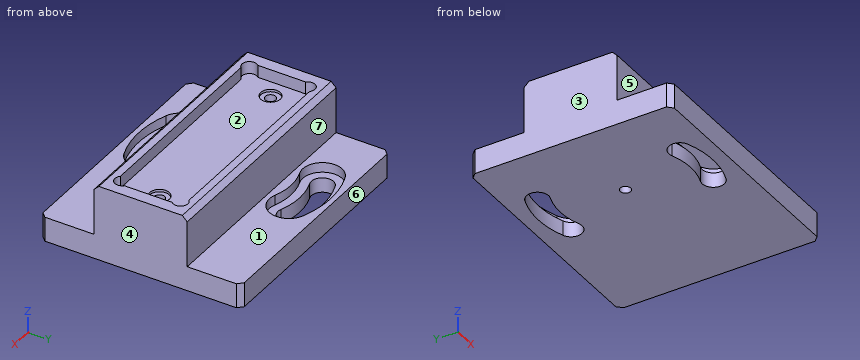
Autodesk Inventor part; units mm, degrees
ref_plane "YZ Plane" through (0, 0, 0) normal (1, 0, 0) x (0, 1, 0)
ref_plane "XZ Plane" through (0, 0, 0) normal (0, 1, 0) x (-1, 0, 0)
ref_plane "XY Plane" through (0, 0, 0) normal (0, 0, 1) x (1, 0, 0)
sketch "Sketch1" plane through (0, 0, 0) normal (0, 0, 1) x (1, 0, 0)
  line L0 (-24.4, -9.5) -> (24.4, -9.5)
  line L1 (24.4, -9.5) -> (24.4, 9.5)
  line L2 (24.4, 9.5) -> (-24.4, 9.5)
  line L3 (-24.4, 9.5) -> (-24.4, -9.5)
  line L4 (-24.4, -9.5) -> (24.4, 9.5) construction
  line L5 (24.4, -9.5) -> (-24.4, 9.5) construction
  point P0 (0, 0)
  dimension "LENGTH" = 48.8
  dimension "WIDTH" = 19
extrude "Extrusion1" add sketch "Sketch1" along normal blind 12.85
sketch "Sketch2" plane through (0, 0, 12.85) normal (0, 0, 1) x (1, 0, 0)
  point P0 (0, 0)
  point P1 (-18.2, 0)
  point P2 (18.2, 0)
  dimension "d11" = 0
  dimension "d12" = 0
  dimension "d13" = 36.4
  dimension "d14" = 18.2
hole "Hole1" at (-18.2, 0, 12.85) at (18.2, 0, 12.85) direction (0, 0, -1) diameter 2.1565 depth 8.87
sketch "Sketch3" plane through (0, 0, 12.85) normal (0, 0, 1) x (1, 0, 0)
  point P0 (0, 0)
  point P1 (0, 0)
  dimension "d22" = 0
  dimension "d23" = 0
hole "Hole2" [suppressed]
sketch "Sketch4" plane through (0, 0, 0) normal (0, 0, -1) x (-1, 0, 0)
  line L0 (5.5, 0) -> (4.5, 0) construction
  line L1 (5.5, 1.05) -> (4.5, 1.05)
  line L2 (4.5, -1.05) -> (5.5, -1.05)
  arc A0 (5.5, -1.05) -> (5.5, 1.05) centre (5.5, 0) ccw
  arc A1 (4.5, 1.05) -> (4.5, -1.05) centre (4.5, 0) ccw
  point P0 (0, 0)
  point P1 (-5, 0)
  point P2 (5, 0)
  dimension "d24" = 1
  dimension "d25" = 0
  dimension "d26" = 0
  dimension "d27" = 10
  dimension "d28" = 5
  dimension "d29" = 1.05
hole "Hole3" [suppressed]
extrude "Extrusion2" [suppressed]
sketch "Sketch5" plane through (0, 0, 0) normal (0, 0, 1) x (1, 0, 0)
  line L0 (-24.4, -20.5) -> (24.4, -20.5)
  line L1 (24.4, -20.5) -> (24.4, 20.5)
  line L2 (24.4, 20.5) -> (-24.4, 20.5)
  line L3 (-24.4, 20.5) -> (-24.4, -20.5)
  line L4 (-24.4, -20.5) -> (24.4, 20.5) construction
  line L5 (24.4, -20.5) -> (-24.4, 20.5) construction
  point P0 (0, 0)
  dimension "d39" = 48.8
  dimension "d40" = 41
extrude "Extrusion3" add sketch "Sketch5" along normal blind 5
sketch "Sketch7" plane through (0, 0, 12.85) normal (0, 0, 1) x (1, 0, 0)
  circle A0 centre (18.2, 0) radius 1.0782
  circle A1 centre (-18.2, 0) radius 1.0782
  point P0 (0, 0)
  dimension "d54" = 0
  dimension "d55" = 0
  dimension "d56" = 0
  dimension "d57" = 0
hole "Hole5" at (18.2, 0, 12.85) at (-18.2, 0, 12.85) direction (0, 0, -1) diameter 4 depth 0.5
chamfer "Chamfer2" distance 1 angle 45 4 edges at (24.4, -20.5, 2.5) (24.4, 20.5, 2.5) (-24.4, 20.5, 2.5) (-24.4, -20.5, 2.5)
sketch "Sketch8" plane through (0, 0, 0) normal (0, 0, -1) x (-1, 0, 0)
  line L0 (0, 5.5) -> (0, 4.5) construction
  line L1 (-1.05, 5.5) -> (-1.05, 4.5)
  line L2 (1.05, 4.5) -> (1.05, 5.5)
  arc A0 (1.05, 5.5) -> (-1.05, 5.5) centre (0, 5.5) ccw
  arc A1 (-1.05, 4.5) -> (1.05, 4.5) centre (0, 4.5) ccw
  point P0 (0, 0)
  point P1 (0, -5)
  point P2 (0, 5)
  dimension "d77" = 1
  dimension "d78" = 1.05
  dimension "d79" = 10
  dimension "d80" = 0
  dimension "d81" = 0
  dimension "d82" = 5
hole "Hole6" [suppressed]
extrude "Extrusion4" [suppressed]
sketch "Sketch9" plane through (-24.4, -19.5, 0) normal (-1, 0, 0) x (0, 0, 1)
  circle A0 centre (-12.35, 19.5) radius 12.7
  line L0 (0, 39) -> (0, 0)
  point P0 (0, 19.5)
  point P1 (0, 16.539)
  point P2 (0, 22.461)
  dimension "d92" = 25.4
  dimension "d93" = 0
  dimension "d94" = 12.35
extrude "Extrusion5" [suppressed]
sketch "Sketch10" plane through (0, 0, 12.85) normal (0, 0, 1) x (1, 0, 0)
  line L0 (-24.4, -9.5) -> (24.4, -9.5)
  line L1 (24.4, -9.5) -> (24.4, 9.5)
  line L2 (24.4, 9.5) -> (-24.4, 9.5)
  line L3 (-24.4, 9.5) -> (-24.4, -9.5)
  line L4 (-24.4, -9.5) -> (24.4, 9.5) construction
  line L5 (24.4, -9.5) -> (-24.4, 9.5) construction
  line L6 (21.9, -7) -> (-21.9, -7)
  line L7 (-21.9, -7) -> (-21.9, 7)
  line L8 (-21.9, 7) -> (21.9, 7)
  line L9 (21.9, 7) -> (21.9, -7)
  line L10 (21.9, -7) -> (-21.9, 7) construction
  line L11 (-21.9, -7) -> (21.9, 7) construction
  circle A0 centre (-20.8393, 5.9393) radius 1.5
  circle A1 centre (-20.8393, -5.9393) radius 1.5
  circle A2 centre (20.8393, 5.9393) radius 1.5
  circle A3 centre (20.8393, -5.9393) radius 1.5
  line L12 (20.8393, 5.9393) -> (21.9, 7)
  line L13 (21.9, -7) -> (20.8393, -5.9393)
  line L14 (-20.8393, 5.9393) -> (-21.9, 7)
  line L15 (-20.8393, -5.9393) -> (-21.9, -7)
  point P0 (0, 0)
  point P1 (21.9, -4.8787)
  point P2 (19.7787, -7)
  point P3 (-19.7787, -7)
  point P4 (-21.9, -4.8787)
  point P5 (-21.9, 4.8787)
  point P6 (-19.7787, 7)
  point P7 (19.7787, 7)
  point P8 (21.9, 4.8787)
  dimension "d106" = 3
  dimension "d110" = 3
  dimension "d111" = 3
  dimension "d112" = 3
  dimension "d97" = 48.8
  dimension "d98" = 19
  dimension "d99" = 43.8
  dimension "d100" = 14
  dimension "d107" = 45
  dimension "d108" = 45
  dimension "d109" = 45
extrude "Extrusion6" add sketch "Sketch10" along normal blind 2.5
chamfer "Chamfer5" [suppressed]
chamfer "Chamfer6" distance 1 angle 45 2 edges at (0, -9.5, 15.35) (0, 9.5, 15.35)
sketch "Sketch12" plane through (0, 0, 5) normal (0, 0, 1) x (1, 0, 0)
  arc A0 (7.9961, 15.4962) -> (-8.004, 14.5013) centre (9.4196, -136.543) ccw construction
  arc A1 (7.9587, 19.496) -> (-8.4624, 18.4749) centre (9.4196, -136.543) ccw
  arc A2 (8.0336, 11.4964) -> (-7.5457, 10.5276) centre (9.4196, -136.543) ccw
  arc A3 (8.0336, 11.4964) -> (7.9587, 19.496) centre (7.9961, 15.4962) ccw
  arc A4 (-8.4624, 18.4749) -> (-7.5457, 10.5276) centre (-8.004, 14.5013) ccw
  line L0 (24.4, 2.961) -> (24.4, -2.961)
  line L1 (24.4, 0) -> (-24.4, 0)
  line L2 (-24.4, 8.5) -> (-24.4, -8.5)
  arc A5 (7.9961, 15.4962) -> (-8.004, 14.5013) centre (9.4196, -136.543) ccw construction
  arc A6 (7.9751, 17.7461) -> (-8.2619, 16.7364) centre (9.4196, -136.543) ccw
  arc A7 (8.0172, 13.2463) -> (-7.7462, 12.2661) centre (9.4196, -136.543) ccw
  arc A8 (8.0172, 13.2463) -> (7.9751, 17.7461) centre (7.9961, 15.4962) ccw
  arc A9 (-8.2619, 16.7364) -> (-7.7462, 12.2661) centre (-8.004, 14.5013) ccw
  arc A10 (-8.004, -14.5013) -> (7.9961, -15.4962) centre (9.4196, 136.543) ccw construction
  arc A11 (-8.4624, -18.4749) -> (7.9587, -19.496) centre (9.4196, 136.543) ccw
  arc A12 (-7.5457, -10.5276) -> (8.0336, -11.4964) centre (9.4196, 136.543) ccw
  arc A13 (7.9587, -19.496) -> (8.0336, -11.4964) centre (7.9961, -15.4962) ccw
  arc A14 (-7.5457, -10.5276) -> (-8.4624, -18.4749) centre (-8.004, -14.5013) ccw
  arc A15 (-8.004, -14.5013) -> (7.9961, -15.4962) centre (9.4196, 136.543) ccw construction
  arc A16 (-8.2619, -16.7364) -> (7.9751, -17.7461) centre (9.4196, 136.543) ccw
  arc A17 (-7.7462, -12.2661) -> (8.0172, -13.2463) centre (9.4196, 136.543) ccw
  arc A18 (7.9751, -17.7461) -> (8.0172, -13.2463) centre (7.9961, -15.4962) ccw
  arc A19 (-7.7462, -12.2661) -> (-8.2619, -16.7364) centre (-8.004, -14.5013) ccw
  point P0 (0, 0)
  point P1 (-8.004, 12.753)
  point P2 (7.9961, 17.2527)
  point P3 (-6.4165, 14.3405)
  point P4 (9.5836, 18.8402)
  point P5 (-8.004, -12.753)
  point P6 (7.9961, -17.2527)
  point P7 (9.5836, -18.8402)
  point P8 (-6.4165, -14.3405)
  dimension "d118" = 8
  dimension "d122" = 4.5
extrude "Extrusion12" [suppressed]
extrude "Extrusion13" [suppressed]
sketch "Sketch14" plane through (0, 0, 0) normal (0, 0, -1) x (-1, 0, 0)
  point P0 (0, 0)
  point P1 (6.4, 0)
hole "Hole7" at (-6.4, 0, 0) direction (0, 0, 1) diameter 2.1 depth 2.1
sketch "Sketch15" plane through (0, 0, 0) normal (0, 0, -1) x (-1, 0, 0)
  circle A0 centre (6.4, 0) radius 1.05
  circle A1 centre (6.4, 0) radius 19.5
  circle A2 centre (6.4, 0) radius 11.5
  circle A3 centre (6.4, 0) radius 17.75
  circle A4 centre (6.4, 0) radius 13.25
  line L0 (-24.4, 9.5) -> (24.4, 9.5)
  line L1 (24.4, 9.5) -> (-24.4, 9.5)
  line L2 (-24.4, -19.5) -> (-24.4, 19.5)
  line L3 (24.4, -9.5) -> (-24.4, -9.5)
  line L4 (24.4, -9.5) -> (-24.4, -9.5)
  arc A5 (9.3371, 17.5053) -> (5.1369, 17.705) centre (6.4, 0) ccw
  arc A6 (8.5925, 13.0673) -> (5.4572, 13.2164) centre (6.4, 0) ccw
  arc A7 (13.9857, 17.9641) -> (-1.4292, 17.8592) centre (6.4, 0) ccw
  arc A8 (10.8736, 10.5942) -> (1.7828, 10.5324) centre (6.4, 0) ccw
  arc A9 (11.8707, 14.5025) -> (0.9294, 14.5025) centre (6.4, 0) ccw construction
  arc A10 (13.2825, 18.2451) -> (-0.4824, 18.2451) centre (6.4, 0) ccw
  arc A11 (10.4589, 10.7599) -> (2.3412, 10.7599) centre (6.4, 0) ccw
  arc A12 (10.4589, 10.7599) -> (13.2825, 18.2451) centre (11.8707, 14.5025) ccw
  arc A13 (-0.4824, 18.2451) -> (2.3412, 10.7599) centre (0.9294, 14.5025) ccw
  arc A14 (11.8707, 14.5025) -> (0.9294, 14.5025) centre (6.4, 0) ccw construction
  arc A15 (12.6648, 16.6077) -> (0.1352, 16.6077) centre (6.4, 0) ccw
  arc A16 (11.0766, 12.3973) -> (1.7235, 12.3973) centre (6.4, 0) ccw
  arc A17 (11.0766, 12.3973) -> (12.6648, 16.6077) centre (11.8707, 14.5025) ccw
  arc A18 (0.1352, 16.6077) -> (1.7235, 12.3973) centre (0.9294, 14.5025) ccw
  line L5 (24.4, 8.5) -> (24.4, -8.5)
  line L6 (24.4, 0) -> (-24.4, 0)
  arc A19 (5.1369, -17.705) -> (9.3371, -17.5053) centre (6.4, 0) ccw
  arc A20 (5.4572, -13.2164) -> (8.5925, -13.0673) centre (6.4, 0) ccw
  arc A21 (-1.4292, -17.8592) -> (13.9857, -17.9641) centre (6.4, 0) ccw
  arc A22 (1.7828, -10.5324) -> (10.8736, -10.5942) centre (6.4, 0) ccw
  arc A23 (0.9294, -14.5025) -> (11.8707, -14.5025) centre (6.4, 0) ccw construction
  arc A24 (-0.4824, -18.2451) -> (13.2825, -18.2451) centre (6.4, 0) ccw
  arc A25 (2.3412, -10.7599) -> (10.4589, -10.7599) centre (6.4, 0) ccw
  arc A26 (13.2825, -18.2451) -> (10.4589, -10.7599) centre (11.8707, -14.5025) ccw
  arc A27 (2.3412, -10.7599) -> (-0.4824, -18.2451) centre (0.9294, -14.5025) ccw
  arc A28 (0.9294, -14.5025) -> (11.8707, -14.5025) centre (6.4, 0) ccw construction
  arc A29 (0.1352, -16.6077) -> (12.6648, -16.6077) centre (6.4, 0) ccw
  arc A30 (1.7235, -12.3973) -> (11.0766, -12.3973) centre (6.4, 0) ccw
  arc A31 (12.6648, -16.6077) -> (11.0766, -12.3973) centre (11.8707, -14.5025) ccw
  arc A32 (1.7235, -12.3973) -> (0.1352, -16.6077) centre (0.9294, -14.5025) ccw
  point P0 (0, 0)
  point P1 (6.4, 15.5)
  point P2 (6.4, -15.5)
  dimension "d140" = 39
  dimension "d141" = 23
  dimension "d142" = 35.5
  dimension "d143" = 26.5
  dimension "d147" = 8
  dimension "d148" = 4.5
sketch "Sketch17" plane through (0, 0, 5) normal (0, 0, 1) x (1, 0, 0)
  circle A0 centre (-6.4, 0) radius 1.05
  arc A1 (-11.8725, -14.4958) -> (-0.9318, -14.4974) centre (-6.4, 0) ccw construction
  arc A2 (-12.6672, -16.6008) -> (-0.1378, -16.6026) centre (-6.4, 0) ccw
  arc A3 (-11.0779, -12.3908) -> (-1.7259, -12.3922) centre (-6.4, 0) ccw
  arc A4 (-11.0779, -12.3908) -> (-12.6672, -16.6008) centre (-11.8725, -14.4958) ccw
  arc A5 (-0.1378, -16.6026) -> (-1.7259, -12.3922) centre (-0.9318, -14.4974) ccw
  arc A6 (-11.8725, -14.4958) -> (-0.9318, -14.4974) centre (-6.4, 0) ccw construction
  arc A7 (-13.2853, -18.238) -> (0.4798, -18.24) centre (-6.4, 0) ccw
  arc A8 (-10.4598, -10.7536) -> (-2.3435, -10.7548) centre (-6.4, 0) ccw
  arc A9 (-10.4598, -10.7536) -> (-13.2853, -18.238) centre (-11.8725, -14.4958) ccw
  arc A10 (0.4798, -18.24) -> (-2.3435, -10.7548) centre (-0.9318, -14.4974) ccw
  line L0 (-24.1444, 0) -> (24.3913, 0)
  line L1 (24.3913, 0) -> (-24.1444, 0)
  arc A11 (-0.9318, 14.4974) -> (-11.8725, 14.4958) centre (-6.4, 0) ccw construction
  arc A12 (-0.1378, 16.6026) -> (-12.6672, 16.6008) centre (-6.4, 0) ccw
  arc A13 (-1.7259, 12.3922) -> (-11.0779, 12.3908) centre (-6.4, 0) ccw
  arc A14 (-12.6672, 16.6008) -> (-11.0779, 12.3908) centre (-11.8725, 14.4958) ccw
  arc A15 (-1.7259, 12.3922) -> (-0.1378, 16.6026) centre (-0.9318, 14.4974) ccw
  arc A16 (-0.9318, 14.4974) -> (-11.8725, 14.4958) centre (-6.4, 0) ccw construction
  arc A17 (0.4798, 18.24) -> (-13.2853, 18.238) centre (-6.4, 0) ccw
  arc A18 (-2.3435, 10.7548) -> (-10.4598, 10.7536) centre (-6.4, 0) ccw
  arc A19 (-13.2853, 18.238) -> (-10.4598, 10.7536) centre (-11.8725, 14.4958) ccw
  arc A20 (-2.3435, 10.7548) -> (0.4798, 18.24) centre (-0.9318, 14.4974) ccw
  point P0 (0, 0)
  point P1 (-0.9324, -14.4958)
  point P2 (-0.9324, 14.4958)
  dimension "d149" = 4.5
  dimension "d150" = 8
extrude "Extrusion14" cut sketch "Sketch17" against normal through all contours A4 A3 A5 A2 | A15 A13 A14 A12
extrude "Extrusion15" cut sketch "Sketch17" against normal blind 2 contours A9 A8 A10 A7 | A20 A18 A19 A17
equation "\"d2\" = BEAM_HEIGHT - APERTURE_HEIGHT"
equation "\"d39\" = LENGTH"
equation "\"d106\" = d110"
equation "\"d111\" = d110"
equation "\"d112\" = d110"
equation "\"d97\" = LENGTH"
equation "\"d98\" = WIDTH"
equation "\"BEAM_HEIGHT\" = 19.05"
equation "\"APERTURE_HEIGHT\" = 6.2"
properties part number "ADAPTER_AOM-brimrose"
The model under review builds one solid part; all positions refer to its coordinate system, in mm. Face numbers are marked on the shaded views. A direction names the side the tool comes from. Coordinates: 2 decimals unless noted, no trailing zeros. Write each loop counter-clockwise with the first axis right and the second up, starting at its lowest first coordinate (ties: lowest second). Pieces come first, ordered by that corner, then holes. Notation, with made-up numbers: (-17, 79.25) - (-5, 79.25) arc R28 cw to (-5, 113.25) - close; hole circle Ø1 at (11.25, 63). An arc over 180 degrees is marked (long way). Answer in a Markdown table with one row per item. Add a question column.
Q1. For the marked faces 5, 6 and 7, list the 3-axis set-ups (+Z, -Z, +X, -X, +Y, -Y) from which the entire face can be reached by the end or side of a thin tool; tool diameter is ignored.
Q2. Consider section D-D on x = 18.2. Give the boundary of the cut face in (y, z).
Q3. Consider section C-C on z = 10.5. Give the boundary of the cut face in (x, y), then the cut area to 3 significant figures.
Q4. Consider section B-B on y = -4. Give the boundary of the cut face in (x, z), then the cut area to 3 significant figures.
Q5. Clearance check with flat-ended pins moving along their axes: pin 1 (2.5 mm diameter, centred on x = -18.5, y = 0.5, fed in from +Z); pin 2 (2.5 mm diameter, centred on x = -10.5, y = 15.5, fed in from +Z); pin 3 (2 mm diameter, centred on x = 6.5, z = 14, fed in from +Y); pin 4 (2 mm diameter, centred on x = 9.5, z = 14.5, fed in from -Y). State where each tip first meets the part, or that it passes through.
Q6. Consider section A-A on x = -6.4. Give the number of separate pieces and of enclosed holes in the cut face, then the cut area to 3 significant figures.
Q7. Draft analysis for pull direction X (two halves, no side actions). For the marked faces 1, 2, 3 and 4, state which applies: +X half, -X half, draft (parallel to the pull), parting line (faces both ways), or undercut.
Q8. To check wall thickness, follow line 1 along X through (y, z) = (0, 12.65); line 2 along X through (y, z) = (0, 9.5); line 3 along Y through (x, z) = (-6.4, 0.55). State the ranges of each line that lie inside material, in increasing order. Write a range as from..to.
Answers below:
| question | item | result |
|---|---|---|
| 1 | face 5 | +Z, +X, -X, -Y |
| 1 | face 6 | +Z, -Z, +X, -X, +Y |
| 1 | face 7 | +Z, +X, -X, +Y |
| 2 | outline | (-20.5, 0) - (20.5, 0) - (20.5, 5) - (9.5, 5) - (9.5, 14.35) - (8.5, 15.35) - (7, 15.35) - (7, 12.85) - (2, 12.85) - (2, 12.35) - (1.08, 12.35) - (1.08, 5) - (-1.08, 5) - (-1.08, 12.35) - (-2, 12.35) - (-2, 12.85) - (-7, 12.85) - (-7, 15.35) - (-8.5, 15.35) - (-9.5, 14.35) - (-9.5, 5) - (-20.5, 5) - close |
| 3 | outline | (-24.4, -9.5) - (24.4, -9.5) - (24.4, 9.5) - (-24.4, 9.5) - close; hole circle Ø2.16 at (-18.2, 0); hole circle Ø2.16 at (18.2, 0) |
| 3 | area | 920 mm² |
| 4 | outline | (-24.4, 0) - (24.4, 0) - (24.4, 15.35) - (21.9, 15.35) - (21.9, 12.85) - (-21.9, 12.85) - (-21.9, 15.35) - (-24.4, 15.35) - close |
| 4 | area | 640 mm² |
| 5 | pin 1 | z = 12.35 |
| 5 | pin 2 | through |
| 5 | pin 3 | y = 9.5 |
| 5 | pin 4 | y = -9.5 |
| 6 | separate pieces | 3 |
| 6 | enclosed holes | 0 |
| 6 | area | 302 mm² |
| 7 | face 1 | draft |
| 7 | face 2 | undercut |
| 7 | face 3 | -X half |
| 7 | face 4 | +X half |
| 8 | line 1 | -24.4..-20.2, -16.2..16.2, 20.2..24.4 |
| 8 | line 2 | -24.4..-19.28, -17.12..17.12, 19.28..24.4 |
| 8 | line 3 | -20.5..-17.74, -13.24..-1.05, 1.05..13.24, 17.74..20.5 |
